Build history of the part. All positions in model axes, mm. Face numbers are marked on the shaded views. A direction names the side the tool comes from. Round coordinates to 2 decimals unless told otherwise and drop trailing zeros. Order: outer loops, then holes, each group sorted by start corner. A loop starts at its lowest first (then second) coordinate and runs counter-clockwise, first axis right, second up. Notation, with made-up numbers: (5, 68) - (47, 68) arc R14 cw to (47, 78) - close; hole circle Ø8 at (82, 7). An arc over 180 degrees is marked (long way). Write each question's results on one line, items separated by ' | '. Start each with the question number.
```python
from build123d import *

# Parameters (mm, degrees)
F0_W           = 45
F0_H           = 75
F1_DEPTH       = 7
F3_D           = 5.5
F3_CBORE_D     = 9.75
F3_CBORE_DEPTH = 5
F4_R           = 4


with BuildPart() as f1:
    # F0 (on Top) → F1 (new body)
    with BuildSketch(Plane.XY):
        Rectangle(F0_W, F0_H)
    extrude(amount=F1_DEPTH)

    # F3 (through all)
    with Locations(Plane.XY.offset(7)):
        with Locations((-9, -24), (9, -24), (9, 24), (-9, 24)):
            CounterBoreHole(F3_D / 2, F3_CBORE_D / 2, F3_CBORE_DEPTH)

    # F4
    f4_edges = [f1.edges().sort_by_distance(p)[0] for p in [
        (22.5, -37.5, 3.5),
        (-22.5, -37.5, 3.5),
        (22.5, 37.5, 3.5),
        (-22.5, 37.5, 3.5),
    ]]
    fillet(f4_edges, radius=F4_R)


solid = f1.part
```
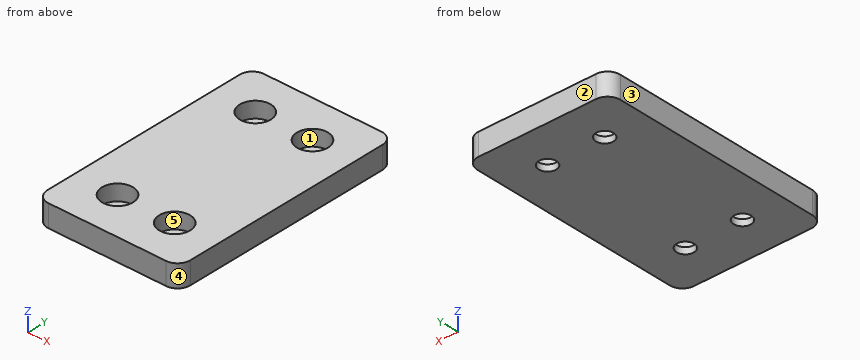
1. Cut at A-A (y = 24). List the corners of the cut face in (x, z) (3 decimals), plus the area to 4 significant figures.
2. Cut at B-B (z = 6.25). List the corners of the cut face in (x, y) (3 decimals), plus the area to 3 significant figures.
3. Flat gauge pins, fed straight in: pin 1 Ø3.5 at (x, y) = (9, -24) entering from +Z; pin 2 Ø9 at (x, y) = (9, 24) entering from +Z. Where does each tip first touch, or does it go through?
4. 3-axis set-ups, long thin cutter, end or side, ignore diameter. For the marked faces 4 and 5: which of +Z, -Z, +X, -X, +Y, -Y reach the whole face in a straight line?
5. Cut at D-D (z = 1.25). List the corners of the cut face in (x, y), plus the area to 3 significant figures.
6. Cut at C-C (x = -9). List the corners of the cut face in (y, z) (3 decimals).
7. Mould opens along X. For the marked faces 1, 2 and 3 say: pulls with the +X half, pulls with the -X half, needs draft (parallel to the pull), parting line crosses it, or undercut.
8. Wall check: line 1 (Y direction, x = -9, z = 1.55); line 2 (Y direction, x = 9, z = 3.6) (3 decimals); line 3 (Z direction, x = 13, y = 23.5). Give the ranges that are in metal, low to high. Write a range as from..to.
A:
1) outline: (-22.5, 0) - (-11.75, 0) - (-11.75, 2) - (-13.875, 2) - (-13.875, 7) - (-22.5, 7) - close; (-6.25, 0) - (6.25, 0) - (6.25, 2) - (4.125, 2) - (4.125, 7) - (-4.125, 7) - (-4.125, 2) - (-6.25, 2) - close; (11.75, 0) - (22.5, 0) - (22.5, 7) - (13.875, 7) - (13.875, 2) - (11.75, 2) - close | area: 195.5 mm^2
2) outline: (-22.5, -33.5) arc R4 ccw to (-18.5, -37.5) - (18.5, -37.5) arc R4 ccw to (22.5, -33.5) - (22.5, 33.5) arc R4 ccw to (18.5, 37.5) - (-18.5, 37.5) arc R4 ccw to (-22.5, 33.5) - close; hole circle Ø9.75 at (-9, -24); hole circle Ø9.75 at (-9, 24); hole circle Ø9.75 at (9, -24); hole circle Ø9.75 at (9, 24) | area: 3,060 mm^2
3) pin 1: passes through | pin 2: stops at z = 2
4) face 4: +Z, -Z, +X, -Y | face 5: +Z
5) outline: (-22.5, -33.5) arc R4 ccw to (-18.5, -37.5) - (18.5, -37.5) arc R4 ccw to (22.5, -33.5) - (22.5, 33.5) arc R4 ccw to (18.5, 37.5) - (-18.5, 37.5) arc R4 ccw to (-22.5, 33.5) - close; hole circle Ø5.5 at (-9, -24); hole circle Ø5.5 at (-9, 24); hole circle Ø5.5 at (9, -24); hole circle Ø5.5 at (9, 24) | area: 3,270 mm^2
6) outline: (-37.5, 0) - (-26.75, 0) - (-26.75, 2) - (-28.875, 2) - (-28.875, 7) - (-37.5, 7) - close; (-21.25, 0) - (21.25, 0) - (21.25, 2) - (19.125, 2) - (19.125, 7) - (-19.125, 7) - (-19.125, 2) - (-21.25, 2) - close; (26.75, 0) - (37.5, 0) - (37.5, 7) - (28.875, 7) - (28.875, 2) - (26.75, 2) - close
7) face 1: undercut | face 2: needs draft | face 3: pulls with the -X half
8) line 1: y = -37.5..-26.75, -21.25..21.25, 26.75..37.5 | line 2: y = -37.5..-28.875, -19.125..19.125, 28.875..37.5 | line 3: z = 0..2
